from build123d import *

# Parameters (mm, degrees)
F0_W     = 25
F0_H     = 25
F0_W_2   = 15
F0_H_2   = 15
F1_DEPTH = 25
F2_W     = 15
F2_H     = 15
F3_DEPTH = 25
F4_W     = 15
F4_H     = 15
F5_DEPTH = 25


with BuildPart() as f1:
    # F0 (on Top) → F1 (new body)
    with BuildSketch(Plane.XY):
        with Locations((8.910105, -12.434757)):
            Rectangle(F0_W, F0_H)
        with Locations((8.910105, -12.434757)):
            Rectangle(F0_W_2, F0_H_2, mode=Mode.SUBTRACT)
    extrude(amount=F1_DEPTH)

    # F2 (on face) → F3 (cut)
    with BuildSketch(Plane.YZ.offset(21.410105)):
        with Locations((-12.434757, 12.5)):
            Rectangle(F2_W, F2_H)
    extrude(amount=-F3_DEPTH, mode=Mode.SUBTRACT)

    # F4 (on face) → F5 (cut)
    with BuildSketch(Plane(origin=(0, 0.065243, 0), x_dir=(-1, 0, 0), z_dir=(0, 1, 0))):
        with Locations((-8.910105, 12.5)):
            Rectangle(F4_W, F4_H)
    extrude(amount=-F5_DEPTH, mode=Mode.SUBTRACT)


solid = f1.part
The model under review builds one solid part; all positions refer to its coordinate system, in mm. A direction names the side the tool comes from. Give positions to 0.01 mm unless a question says otherwise; leave off trailing zeros. Write each loop counter-clockwise with the first axis right and the second up, starting at its lowest first coordinate (ties: lowest second). Pieces come first, ordered by that corner, then holes.
1. Add section C-C, the plane y = -22.25. Write out the cut boundary in (x, z).
2. Draft analysis for pull direction Z (two halves, no side actions). For faces 1 (the flat face through (16.41, -22, 12)), 2 (the flat face through (9, -21, 25)), 3 (the flat face through (9, -4.935, 22)), 4 (the flat face through (-1, -4.935, 12)), state which applies: +Z half, -Z half, draft (parallel to the pull), parting line (faces both ways), or undercut.
3. Add section B-B, the plane z = 6.5. Write out the cut boundary in (x, y).
4. Wall thickness on L1, parallel to Z at x = 9.5, y = -3; L2, parallel to X at y = -4.25, z = 17; L3, parallel to Y at x = 4.5, z = 20.5: over which ranges is each line inside the solid? List them lowest first.
5. Add section A-A, the plane y = -10.25. Write out the cut boundary in (x, z), plus the area to 3 significant figures.
6. For P1, Ø2, axis at x = 1.5, z = 19, coming from the -Y side, flat-tipped, find the tip position at first contact; note if it passes through.
7. Add section D-D, the plane x = -0.75. Write out the cut boundary in (y, z), plus the area to 3 significant figures.
8. Tool access review of faces 5 (the flat face through (9, -4.935, 2)), 6 (the flat face through (19, -19.935, 12)), 7 (the flat face through (9, -2, 20)): name each direction out of +Z, -Z, +X, -X, +Y, -Y from which nothing blocks a thin tool from reaching the whole face with its end or side.
Worked answers:
1. outline: (-3.59, 0) - (21.41, 0) - (21.41, 25) - (-3.59, 25) - close; hole (1.41, 5) - (16.41, 5) - (16.41, 20) - (1.41, 20) - close
2. face 1: undercut
2. face 2: +Z half
2. face 3: draft
2. face 4: undercut
3. outline: (-3.59, -24.93) - (1.41, -24.93) - (1.41, -19.93) - (-3.59, -19.93) - close; (-3.59, -4.93) - (1.41, -4.93) - (1.41, 0.07) - (-3.59, 0.07) - close; (16.41, -24.93) - (21.41, -24.93) - (21.41, -19.93) - (16.41, -19.93) - close; (16.41, -4.93) - (21.41, -4.93) - (21.41, 0.07) - (16.41, 0.07) - close
4. L1: z = 0 to 5, 20 to 25
4. L2: x = -3.59 to 1.41, 16.41 to 21.41
4. L3: y = -24.93 to -19.93, -4.93 to 0.07
5. outline: (-3.59, 0) - (1.41, 0) - (1.41, 5) - (-3.59, 5) - close; (-3.59, 20) - (1.41, 20) - (1.41, 25) - (-3.59, 25) - close; (16.41, 0) - (21.41, 0) - (21.41, 5) - (16.41, 5) - close; (16.41, 20) - (21.41, 20) - (21.41, 25) - (16.41, 25) - close
5. area: 100 mm2
6. P1: stops at y = -24.93
7. outline: (-24.93, 0) - (0.07, 0) - (0.07, 25) - (-24.93, 25) - close; hole (-19.93, 5) - (-4.93, 5) - (-4.93, 20) - (-19.93, 20) - close
7. area: 400 mm2
8. face 5: +Z, -Z
8. face 6: +X, -X
8. face 7: +Y, -Y
